Input: part model. Units: mm. Frame: model coordinates. Face numbers are marked on the shaded views. A direction names the side the tool comes from. Give positions to 0.01 mm unless a question says otherwise; leave off trailing zeros. Write each loop counter-clockwise with the first axis right and the second up, starting at its lowest first coordinate (ties: lowest second). Pieces come first, ordered by that corner, then holes.
```python
from build123d import *

# Parameters (mm, degrees)
EXTRUDE_1_DEPTH     = 8
SKETCH_2_R          = 1.7
CUT_EXTRUDE_1_DEPTH = 8
SKETCH_3_R          = 1.7
CUT_EXTRUDE_2_DEPTH = 8
SKETCH_4_W          = 24
SKETCH_4_H          = 20
EXTRUDE_2_DEPTH     = 5
CHAMFER_1_SIZE      = 2


with BuildPart() as part:
    # 草图1 → 凸台-拉伸1 (new body)
    with BuildSketch(Plane.XY):
        with BuildLine():
            Line((-1.368080573, -3.758770483), (-18.258766079, 2.388936277))
            Line((-18.258766079, 2.388936277), (-48.258766079, 2.388936277))
            Line((-48.258766079, 2.388936277), (-48.258766079, 10.388936277))
            Line((-48.258766079, 10.388936277), (-16.848150233, 10.388936277))
            Line((-16.848150233, 10.388936277), (1.368080573, 3.758770483))
            ThreePointArc((1.368080573, 3.758770483), (3.758770483, -1.368080573), (-1.368080573, -3.758770483))
        make_face()
    extrude(amount=EXTRUDE_1_DEPTH)

    # 草图2 → 切除-拉伸1 (cut)
    with BuildSketch(Plane.XY.offset(8)):
        Circle(SKETCH_2_R)
    extrude(amount=-CUT_EXTRUDE_1_DEPTH, mode=Mode.SUBTRACT)

    # 草图3 → 切除-拉伸2 (cut)
    with BuildSketch(Plane.XY.offset(8)):
        with Locations((-17.553458156, 6.388936277)):
            Circle(SKETCH_3_R)
    extrude(amount=-CUT_EXTRUDE_2_DEPTH, mode=Mode.SUBTRACT)

    # 草图4 → 凸台-拉伸2 (add)
    with BuildSketch(Plane(origin=(0, 10.388936277, 0), x_dir=(1, 0, 0), z_dir=(0, 1, 0))):
        with Locations((-36.258766079, -4)):
            Rectangle(SKETCH_4_W, SKETCH_4_H)
    extrude(amount=-EXTRUDE_2_DEPTH)

    # 倒角1
    chamfer_1_edges = [part.edges().sort_by_distance(p)[0] for p in [
        (-48.258766079, 10.388936277, 4),
    ]]
    chamfer(chamfer_1_edges, length=CHAMFER_1_SIZE)


solid = part.part
```
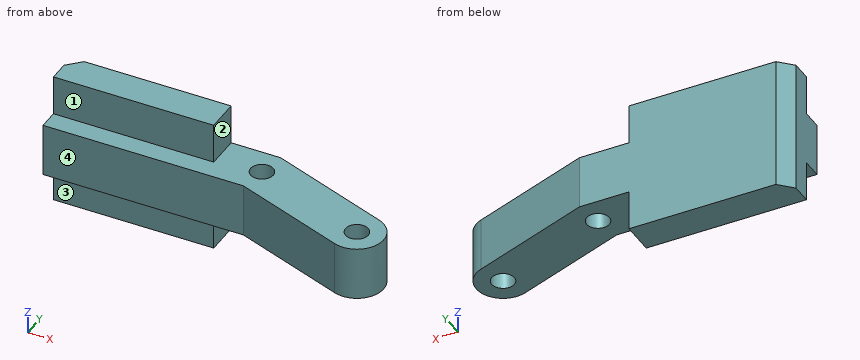
Q1. Section B-B, the plane x = 0. Return the cut outline in (y, z).
Q2. Pin query (flat end, axial travel): pin 1 (4.5 mm diameter, centred on x = -17.55, y = 6.39, fed in from -Z); pin 2 (12 mm diameter, centred on x = -4.5, z = 2.5, fed in from -Y); pin 3 (2 mm diameter, centred on x = 0, y = 0, fed in from +Z); pin 4 (3 mm diameter, centred on x = -37.5, z = 11, fed in from -Y). Return the tip coordinate at first contact, or that it passes through.
Q3. Access query for the marked faces 1, 2, 3 and 4. Directions: +Z, -Z, +X, -X, +Y, -Y. A direction counts if a zero-diameter tool reaches every point of the face in a straight line with its end or side. Return the directions, or none.
Q4. Section A-A, the plane y = -0.5. Return the cut outline in (x, z), then the cut area to 3 significant figures.
Q5. Section C-C, the plane z = 5. Return the cut outline in (x, y).
Q6. Material intervals for line 1 along Z through (x, y) = (-9, 4.5); line 2 along Y through (x, z) = (-25, 13); line 3 along Y through (x, z) = (-26, 5.5), sorted ascending.
Q7. Section D-D, the plane z = -3.5. Return the cut outline in (x, y), then the cut area to 3 significant figures.
Solutions:
1. outline: (-4, 0) - (-1.7, 0) - (-1.7, 8) - (-4, 8) - close; (1.7, 0) - (4.26, 0) - (4.26, 8) - (1.7, 8) - close
2. pin 1: stops at z = 0
2. pin 2: stops at y = -4
2. pin 3: passes through
2. pin 4: stops at y = 5.39
3. face 1: +Z, +X, -X, -Y
3. face 2: +Z, +X, +Y, -Y
3. face 3: -Z, +X, -X, -Y
3. face 4: +Z, -Z, -X, -Y
4. outline: (-10.32, 0) - (-1.62, 0) - (-1.62, 8) - (-10.32, 8) - close; (1.62, 0) - (3.97, 0) - (3.97, 8) - (1.62, 8) - close
4. area: 88.3 mm2
5. outline: (-48.26, 2.39) - (-18.26, 2.39) - (-1.37, -3.76) arc R4 ccw to (1.37, 3.76) - (-16.85, 10.39) - (-46.26, 10.39) - (-48.26, 8.39) - close; hole circle Ø3.4 at (-17.55, 6.39); hole circle Ø3.4 at (0, 0)
6. line 1: z = 0 to 8
6. line 2: y = 5.39 to 10.39
6. line 3: y = 2.39 to 10.39
7. outline: (-48.26, 5.39) - (-24.26, 5.39) - (-24.26, 10.39) - (-46.26, 10.39) - (-48.26, 8.39) - close
7. area: 118 mm2
